from build123d import *

# Parameters (mm, degrees)
SKETCH1_R           = 2
BOSS_EXTRUDE1_DEPTH = 6
CUT_EXTRUDE1_DEPTH  = 3
SKETCH7_R           = 1.984375
CUT_EXTRUDE3_DEPTH  = 6
SKETCH16_W          = 15.013819635
SKETCH16_H          = 6
CUT_EXTRUDE7_DEPTH  = 30.765752132
SKETCH19_R          = 0.5
CUT_EXTRUDE10_DEPTH = 32.527765541
CUT_EXTRUDE13_DEPTH = 3


with BuildPart() as part:
    # Sketch1 → Boss-Extrude1 (new, symmetric)
    with BuildSketch(Plane.XY):
        with BuildLine():
            Line((0, 0), (19, 0))
            ThreePointArc((19, 0), (24.969263034, 5.393453355), (20.206878822, 11.877367056))
            Line((20.206878822, 11.877367056), (5, 15))
            Line((5, 15), (0, 15))
            Line((0, 15), (0, 0))
        make_face()
        with Locations((19, 6)):
            Circle(SKETCH1_R, mode=Mode.SUBTRACT)
    extrude(amount=BOSS_EXTRUDE1_DEPTH, both=True)

    # Sketch2 → Cut-Extrude1 (cut, symmetric)
    with BuildSketch(Plane.XY):
        with BuildLine():
            ThreePointArc((19, 0), (25, 6), (19, 12))
            ThreePointArc((19, 12), (13, 6), (19, 0))
        make_face()
    extrude(amount=CUT_EXTRUDE1_DEPTH, both=True, mode=Mode.SUBTRACT)

    # Sketch7 → Cut-Extrude3 (cut)
    with BuildSketch(Plane.ZY):
        with Locations(Location((-0.32, 10.85, 0), (0, 0, 270))):
            Circle(SKETCH7_R)
        with Locations(Location((-0.32, 4.85, 0), (0, 0, 270))):
            Circle(SKETCH7_R)
    extrude(amount=-CUT_EXTRUDE3_DEPTH, mode=Mode.SUBTRACT)

    # Sketch16 → Cut-Extrude7 (cut, through all)
    with BuildSketch(Plane.XZ):
        with Locations((25.506909818, 0)):
            Rectangle(SKETCH16_W, SKETCH16_H)
    extrude(amount=-CUT_EXTRUDE7_DEPTH, mode=Mode.SUBTRACT)

    # Sketch19 → Cut-Extrude10 (cut, through all)
    with BuildSketch(Plane.XY.offset(6)):
        with Locations((16.5, 3)):
            Circle(SKETCH19_R)
        with Locations((16.5, 9)):
            Circle(SKETCH19_R)
    extrude(amount=-CUT_EXTRUDE10_DEPTH, mode=Mode.SUBTRACT)

    # Sketch23 → Cut-Extrude13 (cut, symmetric)
    with BuildSketch(Plane.XY):
        Polygon((18, 0), (18, 1.5), (16, 1.5), (15, 0), align=None)
    extrude(amount=CUT_EXTRUDE13_DEPTH, both=True, mode=Mode.SUBTRACT)


solid = part.part
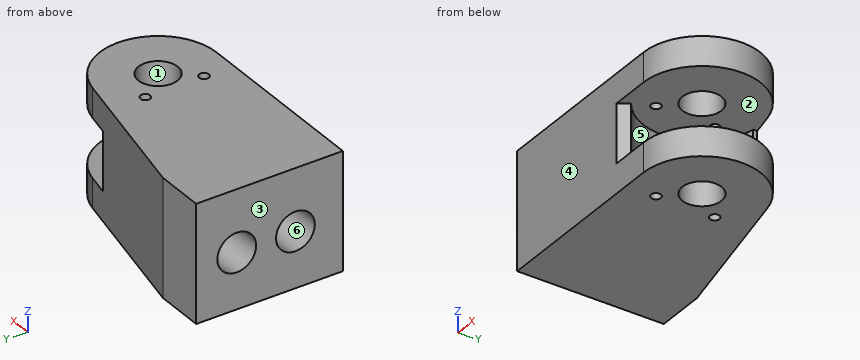
For this review, take the finished solid that the model builds, in its own axes (mm). Face numbers are marked on the shaded views. A direction names the side the tool comes from. Coordinates: 2 decimals unless noted, no trailing zeros. Order: outer loops, then holes, each group sorted by start corner. A loop starts at its lowest first (then second) coordinate and runs counter-clockwise, first axis right, second up. Notation, with made-up numbers: (61, 12) - (89, 12) arc R19 cw to (89, 37) - close; hole circle Ø9 at (29.5, 68.25). An arc over 180 degrees is marked (long way). Use one line per item in the form item = value.
Q1. For the marked faces 4, 5 and 6, list the 3-axis set-ups (+Z, -Z, +X, -X, +Y, -Y) from which the entire face can be reached by the end or side of a thin tool; tool diameter is ignored.
Checked values:
face_4 = +Z, -Z, +X, -X, -Y
face_5 = +X
face_6 = -X
Q2. For P1, Ø4, axis at x = 17, z = 4.5, coming from the +Y side; P2, Ø3, axis at y = 10.85, z = -0.32, coming from the -X side; P3, Ø3, axis at x = 15, z = 4, coming from the +Y side; P4, Ø2.5, axis at x = 19, y = 6, coming from the -Z side, all flat-tipped, find the tip position at first contact; note any pin that passes through.
Checked values:
P1 = 12.95
P2 = 6
P3 = 13.25
P4 = through
Q3. Consider section C-C (y = 6). Give the boundary of the cut face in (x, z), then the cut area to 3 significant figures.
Checked values:
outline = (0, -6) - (17, -6) - (17, -3) - (13, -3) - (13, 3) - (17, 3) - (17, 6) - (0, 6) - (0, 1.3) - (6, 1.3) - (6, -1.94) - (0, -1.94) - close; (21, -6) - (25, -6) - (25, -3) - (21, -3) - close; (21, 3) - (25, 3) - (25, 6) - (21, 6) - close
area = 185 mm2
Q4. Draft analysis for pull direction X (two halves, no side actions). For the marked faces 1, 2 and 3, state which applies: +X half, -X half, draft (parallel to the pull), parting line (faces both ways), or undercut.
Checked values:
face_1 = undercut
face_2 = draft
face_3 = -X half
Q5. Consider section A-A (z = 4.5). Give the boundary of the cut face in (x, y), then the cut area to 3 significant figures.
Checked values:
outline = (0, 0) - (19, 0) arc R6 ccw to (20.21, 11.88) - (5, 15) - (0, 15) - close; hole circle Ø1 at (16.5, 3); hole circle Ø1 at (16.5, 9); hole circle Ø4 at (19, 6)
area = 307 mm2
Q6. For probe 1 along Y at (x, z) = (16.5, 3.7); probe 2 along Z at (x, y) = (3.7, 4.85); probe 3 along X at (y, z) = (6, -4.75), list the stretches that pass through material, from the lowest coordinate up. Write a range as from..to.
Checked values:
probe_1 = 0..2.5, 3.5..8.5, 9.5..12.64
probe_2 = -6..-2.3, 1.66..6
probe_3 = 0..17, 21..25
Q7. Consider section B-B (x = 19.75). Give the boundary of the cut face in (y, z), then the cut area to 3 significant figures.
Checked values:
outline = (0.05, -6) - (4.15, -6) - (4.15, -3) - (0.05, -3) - close; (0.05, 3) - (4.15, 3) - (4.15, 6) - (0.05, 6) - close; (7.85, -6) - (11.97, -6) - (11.97, -3) - (7.85, -3) - close; (7.85, 3) - (11.97, 3) - (11.97, 6) - (7.85, 6) - close
area = 49.3 mm2
Q8. Consider section D-D (x = 16.5). Give the boundary of the cut face in (y, z), then the cut area to 3 significant figures.
Checked values:
outline = (0, -6) - (2.5, -6) - (2.5, -3) - (0, -3) - close; (0, 3) - (2.5, 3) - (2.5, 6) - (0, 6) - close; (3.5, -6) - (8.5, -6) - (8.5, -3) - (3.5, -3) - close; (3.5, 3) - (8.5, 3) - (8.5, 6) - (3.5, 6) - close; (9.5, -6) - (12.64, -6) - (12.64, 6) - (9.5, 6) - (9.5, 3) - (11.45, 3) - (11.45, -3) - (9.5, -3) - close
area = 70.9 mm2
